Can you work these out from the drawing? Everything is in mm from the part's minimum corner. Give positions to 0.01 mm unless a question says otherwise; leave off trailing zeros. Loops run counter-clockwise (first coordinate to the right, second up) from the corner with the lowest first, then second, coordinate; pieces in that order, holes last. Notation, with made-up numbers: (21, 11) -> (72, 11) arc R26 cw to (72, 34) -> close; hole circle Ø9 at (73.5, 83). An arc over 180 degrees is marked (long way). Write item = value, one per line. Start each with the question number.
1) I want a section at B-B (z = 1.85). List the corners of the cut face in (x, y) for me.
2) If we mould it in two halves opening along Z, with no side actions, what happens to the marked faces 1, 2 and 3? For each: +Z half, -Z half, draft (parallel to the pull), parting line (faces both ways), or undercut.
3) I want a section at C-C (y = 2.4). List the corners of the cut face in (x, z) for me (3 decimals), and give its area (3 significant figures).
4) I need wall thicknesses on probe 1 along Z at (x, y) = (1.5, 0.85) (3 decimals); probe 2 along X at (y, z) = (3.1, 1.7); probe 3 along Z at (x, y) = (2.25, 1.8) (3 decimals). Which ranges of each line are inside material? Lowest first, please. Write a range as from..to.
5) I want a section at D-D (z = 3). List the corners of the cut face in (x, y) for me, and give its area (3 significant figures).
6) I want a section at A-A (x = 5). List the corners of the cut face in (y, z) for me (3 decimals), and give its area (3 significant figures).
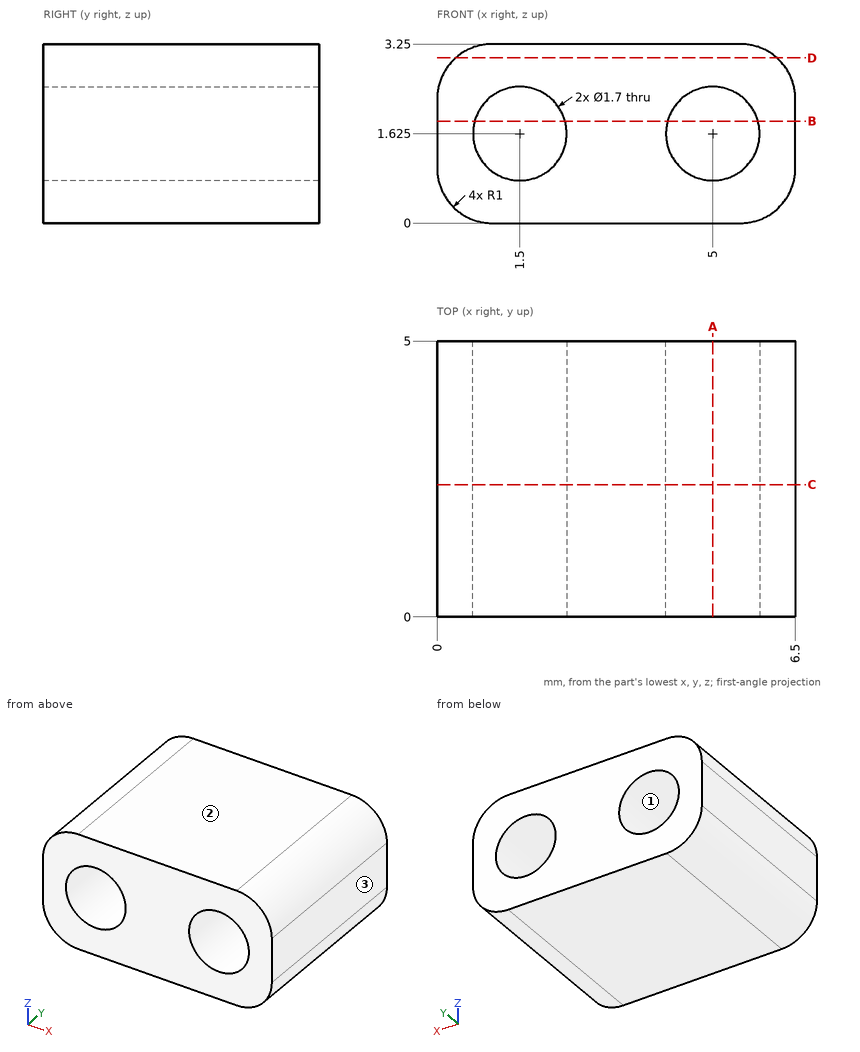
Answer list:
q1.outline = (0, 0) -> (0.68, 0) -> (0.68, 5) -> (0, 5) -> close; (2.32, 0) -> (4.18, 0) -> (4.18, 5) -> (2.32, 5) -> close; (5.82, 0) -> (6.5, 0) -> (6.5, 5) -> (5.82, 5) -> close
q2.face_1 = undercut
q2.face_2 = +Z half
q2.face_3 = draft
q3.outline = (0, 1) arc R1 ccw to (1, 0) -> (5.5, 0) arc R1 ccw to (6.5, 1) -> (6.5, 2.25) arc R1 ccw to (5.5, 3.25) -> (1, 3.25) arc R1 ccw to (0, 2.25) -> close; hole circle Ø1.7 at (1.5, 1.625); hole circle Ø1.7 at (5, 1.625)
q3.area = 15.7 mm^2
q4.probe_1 = 0..0.775, 2.475..3.25
q4.probe_2 = 0..0.65, 2.35..4.15, 5.85..6.5
q4.probe_3 = 0..1.225, 2.025..3.25
q5.outline = (0.34, 0) -> (6.16, 0) -> (6.16, 5) -> (0.34, 5) -> close
q5.area = 29.1 mm^2
q6.outline = (0, 0) -> (5, 0) -> (5, 0.775) -> (0, 0.775) -> close; (0, 2.475) -> (5, 2.475) -> (5, 3.25) -> (0, 3.25) -> close
q6.area = 7.75 mm^2
